Verification items for the finished model (mm, model axes). A direction names the side the tool comes from. Give positions to 0.01 mm unless a question says otherwise; leave off trailing zeros. Loops run counter-clockwise (first coordinate to the right, second up) from the corner with the lowest first, then second, coordinate; pieces in that order, holes last. Notation, with made-up numbers: (70, 86) - (120, 86) arc R16 ccw to (120, 107) - close; hole circle Ø7 at (40, 7). An arc over 180 degrees is marked (long way). One line per item, written item: value. Start each with the question number.
1. Gauge pin test, flat ends, axial feed: pin 1 (1 mm diameter, centred on x = 32.5, y = 1.5, fed in from +Z); pin 2 (5 mm diameter, centred on x = 29.5, y = 6.5, fed in from -Z). Record the tip position at first contact, or that the pin passes through.
2. Scan lines: L1, parallel to X at y = 5.5, z = -15; L2, parallel to X at y = 2, z = -5.5; L3, parallel to X at y = 1.5, z = -27.5. Record each from-to range of solid material in increasing order. Write a range as [from, to].
3. Access from +Z, -Z, +X, -X, +Y, -Y to the whole of each face (thin tool, end or side, straight path). Record for faces 4 (the flat face through (49, 5, -60)), 5 (the flat face through (30, 5, -10)), 6 (the flat face through (30, 5, -37.5)).
4. Sectioned sample at B-B (x = 45). Record the cut outline in (y, z).
5. Sectioned sample at D-D (y = 2.5). Record the cut outline in (x, z), plus the area to 3 significant figures.
6. Sectioned sample at A-A (z = -25). Record the cut outline in (x, y).
7. Mould release check, pull along Z, two halves, no side actions. Record for faces 1 (the flat face through (25, 5, -30)), 2 (the flat face through (22.5, 5, -55)), 3 (the flat face through (11, 5, -60)): pulls with the +Z half, pulls with the -Z half, needs draft (parallel to the pull), parting line crosses it, or undercut.
8. Sectioned sample at C-C (z = -45). Record the cut outline in (x, y).
from build123d import *

# Parameters (mm, degrees)
ESBO_O1_W                = 60
ESBO_O1_H                = 60
RESSALTO_EXTRUS_O1_DEPTH = 10
ESBO_O2_W                = 15
ESBO_O2_H                = 10
CORTE_EXTRUS_O1_DEPTH    = 10
ESBO_O3_W                = 15
ESBO_O3_H                = 10
CORTE_EXTRUS_O2_DEPTH    = 10
ESBO_O4_W                = 10
ESBO_O4_H                = 15
CORTE_EXTRUS_O3_DEPTH    = 86.440037453
ESBO_O5_R                = 1.25
CORTE_EXTRUS_O4_DEPTH    = 86.440037453


with BuildPart() as part:
    # Esboço1 → Ressalto-extrusão1 (new body)
    with BuildSketch(Plane(origin=(0, 0, 0), x_dir=(1, 0, 0), z_dir=(0, 1, 0))):
        with Locations((30, 30)):
            Rectangle(ESBO_O1_W, ESBO_O1_H)
    extrude(amount=RESSALTO_EXTRUS_O1_DEPTH)

    # Esboço2 → Corte-extrusão1 (cut)
    with BuildSketch(Plane.XY):
        with Locations((30, 5)):
            Rectangle(ESBO_O2_W, ESBO_O2_H)
    extrude(amount=-CORTE_EXTRUS_O1_DEPTH, mode=Mode.SUBTRACT)

    # Esboço3 → Corte-extrusão2 (cut)
    with BuildSketch(Plane(origin=(0, 0, -60), x_dir=(-1, 0, 0), z_dir=(0, 0, -1))):
        with Locations((-30, 5)):
            Rectangle(ESBO_O3_W, ESBO_O3_H)
    extrude(amount=-CORTE_EXTRUS_O2_DEPTH, mode=Mode.SUBTRACT)

    # Esboço4 → Corte-extrusão3 (cut, through all)
    with BuildSketch(Plane(origin=(0, 10, 0), x_dir=(1, 0, 0), z_dir=(0, 1, 0))):
        with Locations((30, 30)):
            Rectangle(ESBO_O4_W, ESBO_O4_H)
    extrude(amount=-CORTE_EXTRUS_O3_DEPTH, mode=Mode.SUBTRACT)

    # Esboço5 → Corte-extrusão4 (cut, through all)
    with BuildSketch(Plane(origin=(0, 10, 0), x_dir=(1, 0, 0), z_dir=(0, 1, 0))):
        with Locations(Location((45, 45, 0), (0, 0, 270))):
            Circle(ESBO_O5_R)
        with Locations(Location((15, 45, 0), (0, 0, 270))):
            Circle(ESBO_O5_R)
        with Locations(Location((45, 15, 0), (0, 0, 270))):
            Circle(ESBO_O5_R)
        with Locations(Location((15, 15, 0), (0, 0, 270))):
            Circle(ESBO_O5_R)
    extrude(amount=-CORTE_EXTRUS_O4_DEPTH, mode=Mode.SUBTRACT)


solid = part.part
Results are:
1. pin 1: stops at z = -10
1. pin 2: stops at z = -50
2. L1: x = [0, 13.75], [16.25, 43.75], [46.25, 60]
2. L2: x = [0, 22.5], [37.5, 60]
2. L3: x = [0, 25], [35, 60]
3. face 4: -Z, +X, -X, +Y, -Y
3. face 5: +Z, +Y, -Y
3. face 6: +Y, -Y
4. outline: (0, -60) - (10, -60) - (10, -46.25) - (0, -46.25) - close; (0, -43.75) - (10, -43.75) - (10, -16.25) - (0, -16.25) - close; (0, -13.75) - (10, -13.75) - (10, 0) - (0, 0) - close
5. outline: (0, -60) - (22.5, -60) - (22.5, -50) - (37.5, -50) - (37.5, -60) - (60, -60) - (60, 0) - (37.5, 0) - (37.5, -10) - (22.5, -10) - (22.5, 0) - (0, 0) - close; hole circle Ø2.5 at (15, -45); hole circle Ø2.5 at (15, -15); hole (25, -37.5) - (35, -37.5) - (35, -22.5) - (25, -22.5) - close; hole circle Ø2.5 at (45, -45); hole circle Ø2.5 at (45, -15)
5. area: 3,130 mm^2
6. outline: (0, 0) - (25, 0) - (25, 10) - (0, 10) - close; (35, 0) - (60, 0) - (60, 10) - (35, 10) - close
7. face 1: undercut
7. face 2: needs draft
7. face 3: pulls with the -Z half
8. outline: (0, 0) - (13.75, 0) - (13.75, 10) - (0, 10) - close; (16.25, 0) - (43.75, 0) - (43.75, 10) - (16.25, 10) - close; (46.25, 0) - (60, 0) - (60, 10) - (46.25, 10) - close
